Geometry check sheet. Reference: the model listing, model coordinates, mm. Coordinates: 2 decimals unless noted, no trailing zeros. Write each loop counter-clockwise with the first axis right and the second up, starting at its lowest first coordinate (ties: lowest second). Pieces come first, ordered by that corner, then holes. Notation, with made-up numbers: M 14,66.25 L 71,66.25 A27 ccw 71,99.25 Z; hole C 88.5,41.5 d1. An arc over 180 degrees is marked long. Put each result on its own line as item: value. Start each with the question number.
1) Gauge pin test, flat ends, axial feed: pin 1 (22.5 mm diameter, centred on x = 0, z = 11.5, fed in from +Y); pin 2 (3 mm diameter, centred on y = -2.5, z = 39, fed in from -X); pin 3 (2 mm diameter, centred on x = -6.5, y = -2.5, fed in from +Z); pin 4 (3 mm diameter, centred on y = -2, z = 37.5, fed in from +X). Record the tip position at first contact, or that the pin passes through.
2) Cross-section at A-A on z = 49. Record the cut outline in (x, y).
3) Cross-section at B-B on x = 0. Count the separate pieces of the cut face and the enclosed holes in it, plus the area to 3 significant figures.
4) Scan lines: line 1 along Z through (x, y) = (0, -3.5); line 2 along Z through (x, y) = (-2, -4.25); line 3 along X through (y, z) = (-2.25, 8). Record each from-to range of solid material in increasing order.
5) Mould release check, pull along Z, two halves, no side actions. Record for faces 1 (the cylindrical face through (-23.036, -3.131, -6.108)), 2 (the flat face through (11, 0, 21)): released by +Z, released by -Z, zero draft, split by the parting line, or undercut.
from build123d import *

# Parameters (mm, degrees)
F0_R     = 11.0109
F0_R_2   = 14.1161629055
F1_DEPTH = 6.35


with BuildPart() as f1:
    # F0 (on Front) → F1 (new body)
    with BuildSketch(Plane.XZ):
        with BuildLine():
            add(Edge.make_bspline(
                [(14.2378477878, 44.936459669), (14.2692580265, 44.4830769346), (14.3006366518, 44.0296968618), (14.3328571489, 43.5767591031)],
                knots=[0, 0, 0, 0, 0.0305226673, 0.0305226673, 0.0305226673, 0.0305226673], degree=3))
            ThreePointArc((14.2378477878, 44.936459669), (0.1859137764, 57.5936038827), (-14.1895411716, 45.3051359496))
            add(Edge.make_bspline(
                [(-14.1895411716, 45.3051359496), (-14.2216158391, 45.0234232666), (-14.2536769794, 44.7417099752), (-14.2859418326, 44.4600835103)],
                knots=[0, 0, 0, 0, 0.0190929531, 0.0190929531, 0.0190929531, 0.0190929531], degree=3))
            ThreePointArc((-14.2859418326, 44.4600835103), (-0.6013623419, 28.9346434947), (14.336391997, 43.2584173977))
            ThreePointArc((14.336391997, 43.2584173977), (14.3355082577, 43.4175980628), (14.3328571489, 43.5767591031))
        make_face()
        with Locations((0, 43.2584173977)):
            Circle(F0_R, mode=Mode.SUBTRACT)
        with BuildLine():
            ThreePointArc((14.3328571489, 43.5767591031), (14.3015206028, 44.2577391378), (14.2378477878, 44.936459669))
            add(Edge.make_bspline(
                [(14.2378477878, 44.936459669), (14.2692580265, 44.4830769346), (14.3006366518, 44.0296968618), (14.3328571489, 43.5767591031)],
                knots=[0, 0, 0, 0, 0.0305226673, 0.0305226673, 0.0305226673, 0.0305226673], degree=3))
        make_face()
        with BuildLine():
            add(Edge.make_bspline(
                [(-14.1895411716, 45.3051359496), (-14.2216158391, 45.0234232666), (-14.2536769794, 44.7417099752), (-14.2859418326, 44.4600835103)],
                knots=[0, 0, 0, 0, 0.0190929531, 0.0190929531, 0.0190929531, 0.0190929531], degree=3))
            ThreePointArc((-14.1895411716, 45.3051359496), (-14.2440096703, 44.8833247809), (-14.2859418326, 44.4600835103))
        make_face()
        with BuildLine():
            add(Edge.make_bspline(
                [(14.3328571489, 43.5767591031), (14.8002600895, 37.0062695163), (16.2115652733, 22.8236179544), (31.2555625407, 15.5214679724), (39.4293133759, 11.5620974024)],
                knots=[0.0305226673, 0.0305226673, 0.0305226673, 0.0305226673, 0.4732962362, 1, 1, 1, 1], degree=3))
            ThreePointArc((14.3328571489, 43.5767591031), (14.3355082577, 43.4175980628), (14.336391997, 43.2584173977))
            ThreePointArc((14.336391997, 43.2584173977), (-0.6013623419, 28.9346434947), (-14.2859418326, 44.4600835103))
            add(Edge.make_bspline(
                [(-14.2859418326, 44.4600835103), (-15.0343143138, 37.9278518415), (-16.8442731817, 24.2460870484), (-31.2061924175, 15.6278170074), (-39.061412584, 11.2195897613)],
                knots=[0.0190929531, 0.0190929531, 0.0190929531, 0.0190929531, 0.4619476147, 0.9533331716, 0.9533331716, 0.9533331716, 0.9533331716], degree=3))
            ThreePointArc((-39.061412584, 11.2195897613), (-25.3936507621, 10.1551158407), (-18.8489380989, -1.8909438513))
            ThreePointArc((-18.8489380989, -1.8909438513), (-20.5002656427, -8.5762529664), (-25.0744124588, -13.7238175873))
            add(Edge.make_bspline(
                [(-25.0744124588, -13.7238175873), (-16.8412057321, -11.3905698061), (0.1735884464, -6.5816131812), (18.7761875451, -12.1510294851), (28.3732517974, -15.0335990669)],
                knots=[0, 0, 0, 0, 0.4839699757, 1, 1, 1, 1], degree=3))
            ThreePointArc((28.3732517974, -15.0335990669), (20.9715166849, 3.6392649404), (39.4293133759, 11.5620974024))
        make_face()
        with Locations((0, 11.4961732179)):
            Circle(F0_R_2, mode=Mode.SUBTRACT)
        with BuildLine():
            ThreePointArc((48.6813854206, -1.8909438513), (46.145116247, 6.2727739919), (39.4293133759, 11.5620974024))
            ThreePointArc((39.4293133759, 11.5620974024), (20.9715166849, 3.6392649404), (28.3732517974, -15.0335990669))
            ThreePointArc((28.3732517974, -15.0335990669), (42.1019872984, -13.9858774742), (48.6813854206, -1.8909438513))
        make_face()
        with Locations((34.2746041715, -1.8909438513)):
            Circle(F0_R, mode=Mode.SUBTRACT)
        with BuildLine():
            add(Edge.make_bspline(
                [(-39.061412584, 11.2195897613), (-39.8074219165, 10.8009409398), (-40.5561481429, 10.3834173098), (-41.3048749035, 9.9659258562)],
                knots=[0.9533331716, 0.9533331716, 0.9533331716, 0.9533331716, 1, 1, 1, 1], degree=3))
            ThreePointArc((-39.061412584, 11.2195897613), (-40.2112493235, 10.6430534333), (-41.3048749035, 9.9659258562))
        make_face()
        with BuildLine():
            ThreePointArc((-18.8489380989, -1.8909438513), (-25.3936507621, 10.1551158407), (-39.061412584, 11.2195897613))
            add(Edge.make_bspline(
                [(-39.061412584, 11.2195897613), (-39.8074219165, 10.8009409398), (-40.5561481429, 10.3834173098), (-41.3048749035, 9.9659258562)],
                knots=[0.9533331716, 0.9533331716, 0.9533331716, 0.9533331716, 1, 1, 1, 1], degree=3))
            ThreePointArc((-41.3048749035, 9.9659258562), (-45.0520404312, -10.0061839429), (-25.0744124588, -13.7238175873))
            ThreePointArc((-25.0744124588, -13.7238175873), (-20.5002656427, -8.5762529664), (-18.8489380989, -1.8909438513))
        make_face()
        with Locations((-33.2071557641, -1.8909438513)):
            Circle(F0_R, mode=Mode.SUBTRACT)
    extrude(amount=F1_DEPTH)


solid = f1.part
Answer key:
1. pin 1: passes through
1. pin 2: stops at x = -15.26
1. pin 3: stops at z = 56.5
1. pin 4: stops at x = 15.12
2. outline: M -13.14,-6.35 L -9.4,-6.35 L -9.4,0 L -13.14,0 Z; M 9.4,-6.35 L 13.14,-6.35 L 13.14,0 L 9.4,0 Z
3. separate pieces: 3
3. enclosed holes: 0
3. area: 105 mm²
4. line 1: z = -9.17 to -2.62, 25.61 to 32.25, 54.27 to 57.59
4. line 2: z = -9.19 to -2.48, 25.47 to 32.43, 54.09 to 57.45
4. line 3: x = -43.62 to -38.05, -28.37 to -13.68, 13.68 to 29.44, 39.11 to 44.75
5. face 1: undercut
5. face 2: zero draft
